from build123d import *

# Parameters (mm, degrees)
SKETCH010_W     = 95
SKETCH010_H     = 27
PAD004_DEPTH    = 2
SKETCH011_R     = 1.3
POCKET006_DEPTH = 2
FILLET004_R     = 3
SKETCH012_R     = 1.75
SKETCH012_R_2   = 2.7
POCKET007_DEPTH = 2
SKETCH013_W     = 15.2
SKETCH013_H     = 16.2
SKETCH013_W_2   = 16.4
SKETCH013_H_2   = 13.9
POCKET008_DEPTH = 2


with BuildPart() as part:
    # Sketch010 → Pad004 (new body)
    with BuildSketch(Plane.XY):
        Rectangle(SKETCH010_W, SKETCH010_H)
    extrude(amount=PAD004_DEPTH)

    # Sketch011 (on Face6 of Pad004) → Pocket006 (cut)
    with BuildSketch(Plane.XY.offset(2)):
        with Locations((-44.5, 10.5)):
            Circle(SKETCH011_R)
        with Locations((44.5, 10.5)):
            Circle(SKETCH011_R)
        with Locations((44.5, -10.5)):
            Circle(SKETCH011_R)
        with Locations((-44.5, -10.5)):
            Circle(SKETCH011_R)
    extrude(amount=-POCKET006_DEPTH, mode=Mode.SUBTRACT)

    # Fillet004
    fillet004_edges = [part.edges().sort_by_distance(p)[0] for p in [
        (-47.5, -13.5, 1),
        (47.5, -13.5, 1),
        (47.5, 13.5, 1),
        (-47.5, 13.5, 1),
    ]]
    fillet(fillet004_edges, radius=FILLET004_R)

    # Sketch012 (on Face5 of Fillet004) → Pocket007 (cut)
    with BuildSketch(Plane.XY.offset(2)):
        with Locations((-34.4, -0.3)):
            Circle(SKETCH012_R)
        with Locations((-24.1, 0.3)):
            Circle(SKETCH012_R_2)
    extrude(amount=-POCKET007_DEPTH, mode=Mode.SUBTRACT)

    # Sketch013 (on Face5 of Pocket007) → Pocket008 (cut)
    with BuildSketch(Plane.XY.offset(2)):
        with Locations((12.9, -1.7)):
            Rectangle(SKETCH013_W, SKETCH013_H)
        with Locations((31, -1.7)):
            Rectangle(SKETCH013_W, SKETCH013_H)
        with Locations((-6, -0.55)):
            Rectangle(SKETCH013_W_2, SKETCH013_H_2)
    extrude(amount=-POCKET008_DEPTH, mode=Mode.SUBTRACT)


with BuildPart() as part_1:
    # Body003 placement: moved
    add(part.part.moved(Location((0, -1.2, 135.6))))


solid = part_1.part
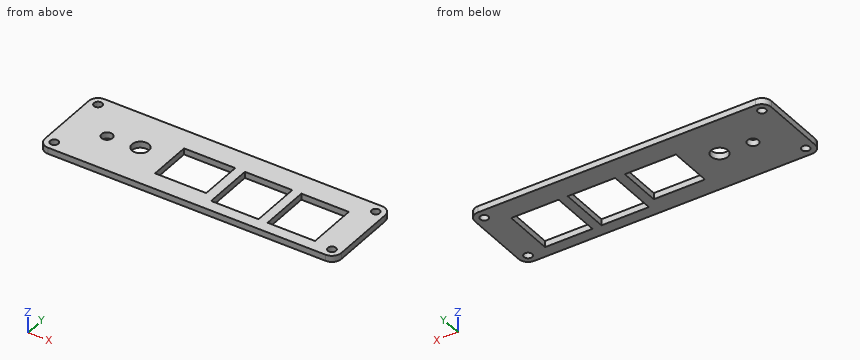
Here's how the part is built. I have some questions about the finished solid (model axes, mm). Coordinates: 2 decimals unless noted, no trailing zeros. Write each loop counter-clockwise with the first axis right and the second up, starting at its lowest first coordinate (ties: lowest second). Pieces come first, ordered by that corner, then holes.
Item 1: I want a section at A-A on x = 36. Write out the boundary of the cut face in (y, z).
Item 2: I want a section at C-C on z = 136.4. Count the separate pieces of the cut face and the enclosed holes in it, and give its area (3 significant figures).
Item 3: I want a section at D-D on x = -24.1. Write out the boundary of the cut face in (y, z).
Item 4: Will this pin go through, and if not, where does the flat tip stop? pin 1 (3 mm diameter, centred on x = -44.5, y = -11.7, fed in from +Z).
Item 5: If I drill on line 1 (X direction, y = -5.25, z = 136.25); line 2 (Y direction, x = -44.5, z = 136.95); line 3 (X direction, y = -9.25, z = 136.7), over which ranges is the centre line in solid material (lowest first)?
Item 6: I want a section at B-B on y = -5. Write out the boundary of the cut face in (x, z), and give its area (3 significant figures).
Findings below:
1. outline: (-14.7, 135.6) - (-11, 135.6) - (-11, 137.6) - (-14.7, 137.6) - close; (5.2, 135.6) - (12.3, 135.6) - (12.3, 137.6) - (5.2, 137.6) - close
2. separate pieces: 1
2. enclosed holes: 9
2. area: 1,780 mm2
3. outline: (-14.7, 135.6) - (-3.6, 135.6) - (-3.6, 137.6) - (-14.7, 137.6) - close; (1.8, 135.6) - (12.3, 135.6) - (12.3, 137.6) - (1.8, 137.6) - close
4. pin 1: stops at z = 137.6
5. line 1: x = -47.5 to -14.2, 2.2 to 5.3, 20.5 to 23.4, 38.6 to 47.5
5. line 2: y = -14.7 to -13, -10.4 to 8, 10.6 to 12.3
5. line 3: x = -47.5 to 5.3, 20.5 to 23.4, 38.6 to 47.5
6. outline: (-47.5, 135.6) - (-14.2, 135.6) - (-14.2, 137.6) - (-47.5, 137.6) - close; (2.2, 135.6) - (5.3, 135.6) - (5.3, 137.6) - (2.2, 137.6) - close; (20.5, 135.6) - (23.4, 135.6) - (23.4, 137.6) - (20.5, 137.6) - close; (38.6, 135.6) - (47.5, 135.6) - (47.5, 137.6) - (38.6, 137.6) - close
6. area: 96.4 mm2
